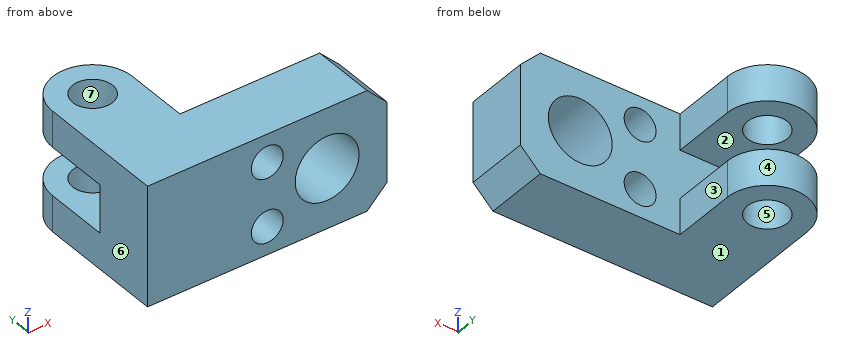
from build123d import *

# Parameters (mm, degrees)
SKETCH2_W           = 60
SKETCH2_H           = 30
BOSS_EXTRUDE1_DEPTH = 16
BOSS_EXTRUDE2_DEPTH = 9
SKETCH4_R           = 5
CUT_EXTRUDE1_DEPTH  = 60.699246226
SKETCH5_R           = 8
SKETCH5_R_2         = 4
CUT_EXTRUDE2_DEPTH  = 43.438190348
CHAMFER1_SIZE       = 5


with BuildPart() as part:
    # Sketch2 → Boss-Extrude1 (new body)
    with BuildSketch(Plane(origin=(0, 0, 0), x_dir=(1, 0, 0), z_dir=(0, 1, 0))):
        Rectangle(SKETCH2_W, SKETCH2_H)
    extrude(amount=BOSS_EXTRUDE1_DEPTH)

    # Sketch3 → Boss-Extrude2 (add)
    with BuildSketch(Plane(origin=(0, 0, -15), x_dir=(-1, 0, 0), z_dir=(0, 0, -1))):
        with BuildLine():
            Line((30, 16), (10, 16))
            Line((10, 16), (10, 32))
            ThreePointArc((10, 32), (20, 42), (30, 32))
            Line((30, 32), (30, 16))
        make_face()
    boss_extrude2 = extrude(amount=-BOSS_EXTRUDE2_DEPTH)

    # Sketch4 → Cut-Extrude1 (cut, through all)
    with BuildSketch(Plane(origin=(0, 0, -15), x_dir=(-1, 0, 0), z_dir=(0, 0, -1))):
        with Locations((20, 32)):
            Circle(SKETCH4_R)
    cut_extrude1 = extrude(amount=-CUT_EXTRUDE1_DEPTH, mode=Mode.SUBTRACT)

    # Mirror1: Boss-Extrude2, Cut-Extrude1 across plane
    add(boss_extrude2.mirror(Plane.XY))
    add(cut_extrude1.mirror(Plane.XY), mode=Mode.SUBTRACT)

    # Sketch5 → Cut-Extrude2 (cut, through all)
    with BuildSketch(Plane(origin=(0, 16, 0), x_dir=(1, 0, 0), z_dir=(0, 1, 0))):
        with Locations(Location((15, 0, 0), (0, 0, 270))):
            Circle(SKETCH5_R)
        with Locations(Location((0, -8, 0), (0, 0, 270))):
            Circle(SKETCH5_R_2)
        with Locations(Location((0, 8, 0), (0, 0, 90))):
            Circle(SKETCH5_R_2)
    extrude(amount=-CUT_EXTRUDE2_DEPTH, mode=Mode.SUBTRACT)

    # Chamfer1
    chamfer1_edges = [part.edges().sort_by_distance(p)[0] for p in [
        (30, 8, 15),
        (30, 8, -15),
    ]]
    chamfer(chamfer1_edges, length=CHAMFER1_SIZE)


solid = part.part
Can you work these out from the model? Positions are in its coordinate system, mm. Face numbers are marked on the shaded views. A direction names the side the tool comes from. Coordinates: 2 decimals unless noted, no trailing zeros. Order: outer loops, then holes, each group sorted by start corner. A loop starts at its lowest first (then second) coordinate and runs counter-clockwise, first axis right, second up. Notation, with made-up numbers: (40, 40.25) -> (74, 40.25) arc R27 cw to (74, 67.25) -> close; hole circle Ø6 at (-1, -35.75). An arc over 180 degrees is marked (long way). Use one line per item in the form item = value.
Q1. Will these pins go through, and if not, where does the flat tip stop? P1, Ø16, axis at x = -20, y = 32, coming from the +Z side; P2, Ø2.5, axis at y = 20.5, z = 11.5, coming from the +X side; P3, Ø12, axis at x = 4.5, z = -8, coming from the +Y side.
From the geometry:
P1 = 15
P2 = -10
P3 = 16
Q2. We'd pull the mould along Y, two halves only. Please class the marked faces 4, 5, 6 and 7: released by +Y, released by -Y, zero draft, split by the parting line, or undercut.
From the geometry:
face_4 = released by +Y
face_5 = undercut
face_6 = zero draft
face_7 = undercut
Q3. Imagine slicing it at D-D, the plane x = 1.5. List the corners of the cut face in (y, z) for me.
From the geometry:
outline = (0, -15) -> (16, -15) -> (16, -11.71) -> (0, -11.71) -> close; (0, -4.29) -> (16, -4.29) -> (16, 4.29) -> (0, 4.29) -> close; (0, 11.71) -> (16, 11.71) -> (16, 15) -> (0, 15) -> close
Q4. Imagine slicing it at C-C, the plane x = 15. List the corners of the cut face in (y, z) for me, then the cut area to 3 significant figures.
From the geometry:
outline = (0, -15) -> (16, -15) -> (16, -8) -> (0, -8) -> close; (0, 8) -> (16, 8) -> (16, 15) -> (0, 15) -> close
area = 224 mm²
Q5. Imagine slicing it at A-A, the plane y = 29. List the corners of the cut face in (x, z) for me.
From the geometry:
outline = (-30, -15) -> (-24, -15) -> (-24, -6) -> (-30, -6) -> close; (-30, 6) -> (-24, 6) -> (-24, 15) -> (-30, 15) -> close; (-16, -15) -> (-10, -15) -> (-10, -6) -> (-16, -6) -> close; (-16, 6) -> (-10, 6) -> (-10, 15) -> (-16, 15) -> close
Q6. Which directions (+Z, -Z, +X, -X, +Y, -Y) give clear straight access to the entire face, cutting with the end or side of a thin tool? Please do the marked faces 1, 2 and 3.
From the geometry:
face_1 = -Z, +X, -X, +Y, -Y
face_2 = +X, -X, +Y
face_3 = +Z, -Z, +X, +Y
Q7. I need wall thicknesses on L1, parallel to Z at x = -26.5, y = 25.5; L2, parallel to Y at x = -20, z = 8.5; L3, parallel to Z at x = -3, y = 14. Which ranges of each line are inside material? Lowest first, please.
From the geometry:
L1 = -15 to -6, 6 to 15
L2 = 0 to 27, 37 to 42
L3 = -15 to -10.65, -5.35 to 5.35, 10.65 to 15
Q8. Imagine slicing it at B-B, the plane z = 0. List the corners of the cut face in (x, y) for me.
From the geometry:
outline = (-30, 0) -> (7, 0) -> (7, 16) -> (-30, 16) -> close; (23, 0) -> (30, 0) -> (30, 16) -> (23, 16) -> close
